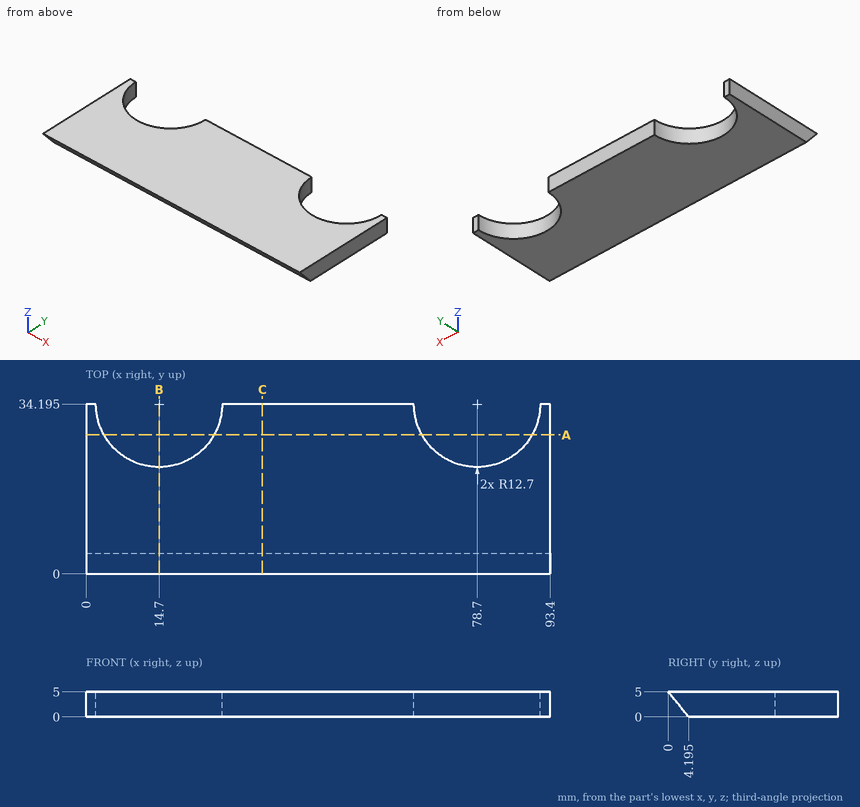
Can you work these out from the drawing? Everything is in mm from the part's minimum corner. Coordinates: 2 decimals unless noted, no trailing zeros. Loops run counter-clockwise (first coordinate to the right, second up) from the corner with the lowest first, then second, coordinate; pieces in that order, holes last.
1. Imagine slicing it at C-C, the plane x = 35.5. Please give me the cut outline in (y, z) (1 decimal).
2. Imagine slicing it at B-B, the plane x = 14.7. Please give me the cut outline in (y, z) (1 decimal).
3. For P1, Ø5, axis at x = 70.5, y = 10, coming from the -Z side; P2, Ø3, axis at x = 73, z = 4, coming from the +Y side (1 decimal), each with a flat end and sliding along its axis, tell me the tip position at first contact or that it passes through.
4. I need wall thicknesses on L1, parallel to X at y = 30, z = 0.95; L2, parallel to X at y = 26, z = 2.65; L3, parallel to Z at x = 54, y = 3.5. Which ranges of each line are inside material? Lowest first, please.
5. Imagine slicing it at A-A, the plane y = 28. Please give me the cut outline in (x, z).
Taken from the geometry:
1. outline: (0, 5) - (4.2, 0) - (34.2, 0) - (34.2, 5) - close
2. outline: (0, 5) - (4.2, 0) - (21.5, 0) - (21.5, 5) - close
3. P1: stops at z = 0
3. P2: stops at y = 23.7
4. L1: x = 0 to 2.71, 26.69 to 66.71, 90.69 to 93.4
4. L2: x = 0 to 5, 24.4 to 69, 88.4 to 93.4
4. L3: z = 0.83 to 5
5. outline: (0, 0) - (3.61, 0) - (3.61, 5) - (0, 5) - close; (25.79, 0) - (67.61, 0) - (67.61, 5) - (25.79, 5) - close; (89.79, 0) - (93.4, 0) - (93.4, 5) - (89.79, 5) - close
